from build123d import *

# Parameters (mm, degrees)
F0_R     = 12.7
F1_DEPTH = 76.2
F3_R     = 12.7
F3_R_2   = 6.35
F4_DEPTH = 63.246
F5_R     = 2.1129626077
F6_DEPTH = 12.7


# Not quite as in the source:
# - a fillet or chamfer that OpenCascade refuses, or shapes differently, is made with other operations: its cross-section is extruded or revolved along the edge and cut away or added


with BuildPart() as f1:
    # F0 (on Front) → F1 (new body)
    with BuildSketch(Plane.XZ):
        Circle(F0_R)
    extrude(amount=F1_DEPTH)

    # F2: fillet of radius 12.7 on 1 edges, made by hand

    # F2_s1 → F2_t2 (revolve, cut)
    with BuildSketch(Plane.XY):
        with BuildLine():
            add(Edge.make_bspline(
                [(12.7, -63.5), (12.7, -76.2), (0, -76.2)],
                knots=[0, 0, 0, 1, 1, 1], degree=2, weights=[1, 0.1764705882, 1]))
            Line((0, -76.2), (12.7, -76.2))
            Line((12.7, -76.2), (12.7, -63.5))
        make_face()
    revolve(axis=Axis((0, -76.2, 0), (0, -1, 0)), mode=Mode.SUBTRACT)

    # F3 (on face) → F4 (cut)
    with BuildSketch(Plane(origin=(0, 0, 0), x_dir=(-1, 0, 0), z_dir=(0, 1, 0))):
        Circle(F3_R)
        Circle(F3_R_2, mode=Mode.SUBTRACT)
    extrude(amount=-F4_DEPTH, mode=Mode.SUBTRACT)

    # F5 (on face) → F6 (cut)
    with BuildSketch(Plane(origin=(0, 0, 0), x_dir=(-1, 0, 0), z_dir=(0, 1, 0))):
        Circle(F5_R)
    extrude(amount=-F6_DEPTH, mode=Mode.SUBTRACT)


solid = f1.part
Could you check a few things on this model? Use its own coordinates, in mm. Round coordinates to 2 decimals unless told otherwise and drop trailing zeros. Write each loop counter-clockwise with the first axis right and the second up, starting at its lowest first coordinate (ties: lowest second). Pieces come first, ordered by that corner, then holes. Notation, with made-up numbers: (65, -20) -> (123, -20) arc R10 ccw to (123, -11) -> close; hole circle Ø3 at (25, 15.5). An arc over 180 degrees is marked (long way). Use a Markdown table: item, result.
1. We'd pull the mould along Z, two halves only. Please class faces 1 (the face through (1.38, -31.18, -6.2)), 2 (the face through (1.677, -6.261, -1.286)), 3 (the face through (-2, 0, 2)): +Z half, -Z half, draft (parallel to the pull), parting line (faces both ways), or undercut.
Answer key:
| item | result |
|---|---|
| face 1 | parting line |
| face 2 | undercut |
| face 3 | draft |
2. For pin 1 Ø5 at (x, y) = (-4, -17.5) entering from -Z; pin 2 Ø8 at (x, z) = (-4.5, -9) entering from -Y; pin 3 Ø2 at (x, z) = (0, 1) entering from +Y, each with a flat end and sliding along its axis, tell me the tip position at first contact or that it passes through.
Answer key:
| item | result |
|---|---|
| pin 1 | stops at z = -6.17 |
| pin 2 | stops at y = -72 |
| pin 3 | stops at y = -12.7 |
3. Please list where these lines run through material, in increasing order: probe 1 along Z at (x, y) = (0, -6.25); probe 2 along X at (y, z) = (-6, -5.5); probe 3 along Y at (x, z) = (11.75, 2.5).
Answer key:
| item | result |
|---|---|
| probe 1 | z = -6.35 to -2.11, 2.11 to 6.35 |
| probe 2 | x = -3.17 to 3.17 |
| probe 3 | y = -65.16 to -63.25 |
4. If we section it at A-A (y = -28): List the corners of the cut face in (x, z) for me.
Answer key:
| item | result |
|---|---|
| outline | circle Ø12.7 at (0, 0) |
